Source: CAD feature listing. Evaluate the final solid. Frame: model axes, mm. Face numbers are marked on the shaded views. A direction names the side the tool comes from. Coordinates: 2 decimals unless noted, no trailing zeros. Write each loop counter-clockwise with the first axis right and the second up, starting at its lowest first coordinate (ties: lowest second). Pieces come first, ordered by that corner, then holes. Notation, with made-up numbers: (-1.75, -9.5) - (57.25, -9.5) arc R22 ccw to (57.25, 3.5) - close; hole circle Ø2 at (73.5, 25). An arc over 180 degrees is marked (long way). One line per item, written item: value.
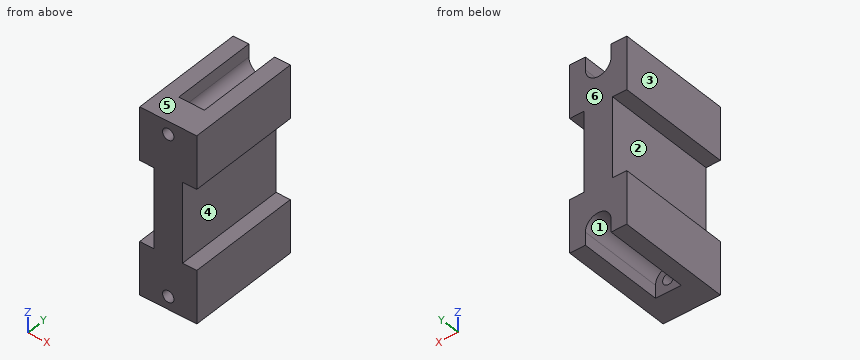
from build123d import *

# Parameters (mm, degrees)
SKETCH1_W           = 20
SKETCH1_H           = 65
BOSS_EXTRUDE1_DEPTH = 40
SKETCH2_R           = 2
SKETCH2_W           = 5
SKETCH2_H           = 28
CUT_EXTRUDE1_DEPTH  = 40
SKETCH4_R           = 4.5
SKETCH4_W           = 9
SKETCH4_H           = 4.5
CUT_EXTRUDE4_DEPTH  = 30


with BuildPart() as part:
    # Sketch1 → Boss-Extrude1 (new body)
    with BuildSketch(Plane(origin=(0, 0, 0), x_dir=(1, 0, 0), z_dir=(0, 1, 0))):
        with Locations((10, 32.5)):
            Rectangle(SKETCH1_W, SKETCH1_H)
    extrude(amount=BOSS_EXTRUDE1_DEPTH)

    # Sketch2 → Cut-Extrude1 (cut)
    with BuildSketch(Plane(origin=(0, 40, 0), x_dir=(1, 0, 0), z_dir=(0, 1, 0))):
        with Locations((10, 60.5)):
            Circle(SKETCH2_R)
        with Locations((10, 4.5)):
            Circle(SKETCH2_R)
        with Locations((17.5, 32.5)):
            Rectangle(SKETCH2_W, SKETCH2_H)
        with Locations((2.5, 32.5)):
            Rectangle(SKETCH2_W, SKETCH2_H)
    extrude(amount=-CUT_EXTRUDE1_DEPTH, mode=Mode.SUBTRACT)

    # Sketch4 → Cut-Extrude4 (cut)
    with BuildSketch(Plane(origin=(0, 40, 0), x_dir=(1, 0, 0), z_dir=(0, 1, 0))):
        with Locations((10, 4.5)):
            Circle(SKETCH4_R)
        with Locations((10, 60.5)):
            Circle(SKETCH4_R)
        with Locations((10, 2.25)):
            Rectangle(SKETCH4_W, SKETCH4_H)
        with Locations((10, 62.75)):
            Rectangle(SKETCH4_W, SKETCH4_H)
    extrude(amount=-CUT_EXTRUDE4_DEPTH, mode=Mode.SUBTRACT)


solid = part.part
1) Contact query for flat-ended pins moving along their axis: P1, Ø8, axis at y = 34.5, z = -20, coming from the -X side; P2, Ø8.5, axis at y = 14.5, z = -28, coming from the +X side; P3, Ø4, axis at y = 34.5, z = -39, coming from the -X side; P4, Ø5, axis at x = 10, z = -60.5, coming from the +Y side. Output: stop coordinate, or through.
Values found:
P1: x = 0
P2: x = 15
P3: x = 5
P4: y = 10
2) Reachability of the marked faces 1, 2 and 3 from +Z, -Z, +X, -X, +Y, -Y: full face, straight path, thin tool, end or side. Return the list, or none.
Values found:
face 1: -Z, +Y
face 2: -X, +Y, -Y
face 3: +Z, -Z, -X, +Y, -Y
3) Section query C-C on y = 35. Output: boundary loops of the cut face in (x, z).
Values found:
outline: (0, -65) - (5.5, -65) - (5.5, -60.5) arc R4.5 cw to (14.5, -60.5) - (14.5, -65) - (20, -65) - (20, -46.5) - (15, -46.5) - (15, -18.5) - (20, -18.5) - (20, 0) - (14.5, 0) - (14.5, -4.5) arc R4.5 cw to (5.5, -4.5) - (5.5, 0) - (0, 0) - (0, -18.5) - (5, -18.5) - (5, -46.5) - (0, -46.5) - close
4) Section query D-D on z = -27.5. Output: boundary loops of the cut face in (x, y), then the cut area to 3 significant figures.
Values found:
outline: (5, 0) - (15, 0) - (15, 40) - (5, 40) - close
area: 400 mm2
5) Section query B-B on x = 10. Output: boundary loops of the cut face in (y, z), then the cut area to 3 significant figures.
Values found:
outline: (0, -65) - (10, -65) - (10, -62.5) - (0, -62.5) - close; (0, -58.5) - (10, -58.5) - (10, -56) - (40, -56) - (40, -9) - (10, -9) - (10, -6.5) - (0, -6.5) - close; (0, -2.5) - (10, -2.5) - (10, 0) - (0, 0) - close
area: 1,980 mm2
6) Section query A-A on x = 16.25. Output: boundary loops of the cut face in (y, z).
Values found:
outline: (0, -65) - (40, -65) - (40, -46.5) - (0, -46.5) - close; (0, -18.5) - (40, -18.5) - (40, 0) - (0, 0) - close
7) Draft query along Z for the marked faces 4, 5 and 6. Return one class per face: released by +Z, released by -Z, zero draft, split by the parting line, or undercut.
Values found:
face 4: undercut
face 5: released by +Z
face 6: zero draft
8) Material intervals for line 1 (Z direction, x = 10, y = 7.5); line 2 (Z direction, x = 4.5, y = 20.5); line 3 (Z direction, x = 8.5, y = 6.5), sorted ascending.
Values found:
line 1: -65 to -62.5, -58.5 to -6.5, -2.5 to 0
line 2: -65 to -46.5, -18.5 to 0
line 3: -65 to -61.82, -59.18 to -5.82, -3.18 to 0
